```python
from build123d import *

# Parameters (mm, degrees)
BOSS_EXTRUDE2_DEPTH = 10
FILLET1_R           = 5
FILLET2_R           = 1
SKETCH2_R           = 2.6
CUT_EXTRUDE1_DEPTH  = 46.191260217


with BuildPart() as part:
    # Sketch1 → Boss-Extrude2 (new body)
    with BuildSketch(Plane.XY):
        Polygon((-18.5, -10.2), (-18.5, -20), (18.5, -20), (18.5, -10.2), (4.5, -10.2), (4.5, 10.2), (18.5, 10.2), (18.5, 20), (-18.5, 20), (-18.5, 10.2), (-4.5, 10.2), (-4.5, -10.2), align=None)
    extrude(amount=BOSS_EXTRUDE2_DEPTH)

    # Fillet1
    fillet1_edges = [part.edges().sort_by_distance(p)[0] for p in [
        (18.5, 15.1, 0),
        (18.5, 15.1, 10),
        (18.5, -15.1, 0),
        (18.5, -15.1, 10),
        (-18.5, 15.1, 0),
        (-18.5, -15.1, 0),
        (-18.5, -15.1, 10),
        (-18.5, 15.1, 10),
    ]]
    fillet(fillet1_edges, radius=FILLET1_R - 0.0001)  # a hair under: the kernel refuses the full size

    # Fillet2
    fillet2_edges = [part.edges().sort_by_distance(p)[0] for p in [
        (4.5, 0, 10),
        (-4.5, 0, 0),
        (4.5, 0, 0),
        (-4.5, 0, 10),
    ]]
    fillet(fillet2_edges, radius=FILLET2_R)

    # Sketch2 → Cut-Extrude1 (cut, through all)
    with BuildSketch(Plane.XZ.offset(20)):
        with Locations(Location((-13.5, 5, 0), (0, 0, 270))):
            Circle(SKETCH2_R)
        with Locations(Location((13.5, 5, 0), (0, 0, 270))):
            Circle(SKETCH2_R)
    extrude(amount=-CUT_EXTRUDE1_DEPTH, mode=Mode.SUBTRACT)


solid = part.part
```
Verification items for the finished model (mm, model axes). A direction names the side the tool comes from. Give positions to 0.01 mm unless a question says otherwise; leave off trailing zeros. Order: outer loops, then holes, each group sorted by start corner. A loop starts at its lowest first (then second) coordinate and runs counter-clockwise, first axis right, second up. Notation, with made-up numbers: (62.5, 74) -> (88.5, 74) arc R24 cw to (88.5, 90) -> close; hole circle Ø7 at (41.25, 79.5). An arc over 180 degrees is marked (long way). Use a Markdown table: item, result.
1) Section check A-A, the plane y = 16. Give the number of separate pieces and of enclosed holes in the cut face, then the cut area to 3 significant figures.
Results:
| item | result |
|---|---|
| separate pieces | 1 |
| enclosed holes | 2 |
| area | 306 mm² |
2) Mould release check, pull along Y, two halves, no side actions. Record for faces 1 (the flat face through (10.9, 10.2, 6)), 2 (the flat face through (0, 20, 5)), 3 (the cylindrical face through (-17.07, 15.03, 8.5)): pulls with the +Y half, pulls with the -Y half, needs draft (parallel to the pull), parting line crosses it, or undercut.
Results:
| item | result |
|---|---|
| face 1 | undercut |
| face 2 | pulls with the +Y half |
| face 3 | needs draft |
3) Section check D-D, the plane y = -6. Record the boundary of the cut face in (x, z).
Results:
| item | result |
|---|---|
| outline | (-4.5, 1) arc R1 ccw to (-3.5, 0) -> (3.5, 0) arc R1 ccw to (4.5, 1) -> (4.5, 9) arc R1 ccw to (3.5, 10) -> (-3.5, 10) arc R1 ccw to (-4.5, 9) -> close |
4) Tool access check on faces 4 (the cylindrical face through (-4.199, -0.143, 0.285)), 5 (the cylindrical face through (4.199, 0.143, 9.715)), 6 (the cylindrical face through (4.199, 0.143, 0.285)), 7 (the flat face through (4.5, 0, 5)). Record the directions out of +Z, -Z, +X, -X, +Y, -Y that give a thin tool (end or side, any length) a straight path to the whole face; none if there is none.
Results:
| item | result |
|---|---|
| face 4 | -Z, -X |
| face 5 | +Z, +X |
| face 6 | -Z, +X |
| face 7 | +Z, -Z, +X |
5) Section check B-B, the plane z = 4.25. Record the boundary of the cut face in (x, y), then the cut area to 3 significant figures.
Results:
| item | result |
|---|---|
| outline | (-18.44, -20) -> (-15.99, -20) -> (-15.99, -10.2) -> (-18.44, -10.2) -> close; (-18.44, 10.2) -> (-15.99, 10.2) -> (-15.99, 20) -> (-18.44, 20) -> close; (-11.01, -20) -> (11.01, -20) -> (11.01, -10.2) -> (4.5, -10.2) -> (4.5, 10.2) -> (11.01, 10.2) -> (11.01, 20) -> (-11.01, 20) -> (-11.01, 10.2) -> (-4.5, 10.2) -> (-4.5, -10.2) -> (-11.01, -10.2) -> close; (15.99, -20) -> (18.44, -20) -> (18.44, -10.2) -> (15.99, -10.2) -> close; (15.99, 10.2) -> (18.44, 10.2) -> (18.44, 20) -> (15.99, 20) -> close |
| area | 711 mm² |
6) Depth check by flat-ended pin: pin 1 Ø4.5 at (x, z) = (13.5, 5) entering from -Y; pin 2 Ø5 at (x, z) = (-11.5, 3.5) entering from -Y; pin 3 Ø5 at (y, z) = (7, 2) entering from -X. Enter the tip coordinate at first touch or a pass-through.
Results:
| item | result |
|---|---|
| pin 1 | through |
| pin 2 | y = -20 |
| pin 3 | x = -4.5 |
7) Material ranges on probe 1 along X at (y, z) = (17, 5); probe 2 along Y at (x, z) = (-14, 8.75); probe 3 along X at (y, z) = (13.5, 2.75), recorded low to high.
Results:
| item | result |
|---|---|
| probe 1 | -18.5 to -16.1, -10.9 to 10.9, 16.1 to 18.5 |
| probe 2 | -20 to -10.2, 10.2 to 20 |
| probe 3 | -17.97 to -14.8, -12.2 to 12.2, 14.8 to 17.97 |
8) Section check C-C, the plane x = 10. Record the boundary of the cut face in (y, z).
Results:
| item | result |
|---|---|
| outline | (-20, 0) -> (-10.2, 0) -> (-10.2, 10) -> (-20, 10) -> close; (10.2, 0) -> (20, 0) -> (20, 10) -> (10.2, 10) -> close |
